Could you check a few things on this model? Use its own coordinates, in mm. A direction names the side the tool comes from. Coordinates: 2 decimals unless noted, no trailing zeros. Loops run counter-clockwise (first coordinate to the right, second up) from the corner with the lowest first, then second, coordinate; pieces in that order, holes last.
1) Imagine slicing it at B-B on x = -11.25. Please give me the cut outline in (y, z) (3 decimals).
2) Will these pins go through, and if not, where does the flat tip stop? P1, Ø8, axis at y = 51, z = 36, coming from the +X side; P2, Ø3, axis at y = 14, z = 65.5, coming from the -X side; P3, Ø8, axis at y = 56.5, z = 43, coming from the +X side.
3) If I drill on line 1 along Y through (x, z) = (-6.75, 43); line 2 along Y through (x, z) = (2.25, 12.5); line 3 along Y through (x, z) = (-6.5, 71), over which ranges is the centre line in solid material (lowest first)?
4) Imagine slicing it at A-A on y = 58. Please give me the cut outline in (x, z), plus the area to 3 significant figures.
5) Imagine slicing it at C-C on y = 26. Give the number of separate pieces and of enclosed holes in the cut face, plus the area to 3 significant figures.
6) For faces 3 (the face through (3.048, 25, 37)), 4 (the face through (-2, 19, 57.023)), which set-ups out of +Z, -Z, +X, -X, +Y, -Y let a thin tool reach every point of the face, with its end or its side?
7) Thinking about a two-plate mould opening in Z: for faces 1 (the face through (-2, 19, 2.159)), 2 (the face through (2, 0, 55)), which applies, released by +Z, released by -Z, zero draft, split by the parting line, or undercut?
```python
from build123d import *

# Parameters (mm, degrees)
BOSS_EXTRUDE1_DEPTH = 75.184
FILLET1_R           = 6.35
SKETCH6_R           = 3.175
CUT_EXTRUDE2_DEPTH  = 62.992
SKETCH11_W          = 5.969
SKETCH11_H          = 31.75
CUT_EXTRUDE6_DEPTH  = 100.663851822


with BuildPart() as part:
    # Sketch1 → Boss-Extrude1 (new body)
    with BuildSketch(Plane.XY):
        Polygon((0, 0), (3.048, 0), (3.048, 41.91), (-6.35, 47.752), (-6.35, 63.5), (-12.7, 63.5), (-12.7, 40.64), align=None)
    extrude(amount=BOSS_EXTRUDE1_DEPTH)

    # Fillet1
    fillet1_edges = [part.edges().sort_by_distance(p)[0] for p in [
        (-9.525, 63.5, 75.184),
        (-9.525, 63.5, 0),
    ]]
    fillet(fillet1_edges, radius=FILLET1_R)

    # Sketch6 → Cut-Extrude2 (cut, symmetric)
    with BuildSketch(Plane(origin=(-6.35, 0, 0), x_dir=(0, 0, -1), z_dir=(1, 0, 0))):
        with Locations(Location((-68.834, 57.15, 0), (0, 0, 90))):
            Circle(SKETCH6_R)
        with Locations(Location((-6.35, 57.15, 0), (0, 0, 90))):
            Circle(SKETCH6_R)
    extrude(amount=CUT_EXTRUDE2_DEPTH, both=True, mode=Mode.SUBTRACT)

    # Sketch11 → Cut-Extrude6 (cut, through all)
    with BuildSketch(Plane(origin=(3.048, 0, 0), x_dir=(0, 0, -1), z_dir=(1, 0, 0))):
        with Locations((-69.1515, 15.875)):
            Rectangle(SKETCH11_W, SKETCH11_H)
        with Locations((-60.0075, 15.875)):
            Rectangle(SKETCH11_W, SKETCH11_H)
        with Locations((-50.8635, 15.875)):
            Rectangle(SKETCH11_W, SKETCH11_H)
        with Locations((-41.7195, 15.875)):
            Rectangle(SKETCH11_W, SKETCH11_H)
        with Locations((-32.5755, 15.875)):
            Rectangle(SKETCH11_W, SKETCH11_H)
        with Locations((-23.4315, 15.875)):
            Rectangle(SKETCH11_W, SKETCH11_H)
        with Locations((-14.2875, 15.875)):
            Rectangle(SKETCH11_W, SKETCH11_H)
        with Locations((-5.1435, 15.875)):
            Rectangle(SKETCH11_W, SKETCH11_H)
    extrude(amount=-CUT_EXTRUDE6_DEPTH, mode=Mode.SUBTRACT)


solid = part.part
```
Filled in:
1. outline: (36, 0) - (57.15, 0) arc R6.35 ccw to (63.5, 6.35) - (63.5, 68.834) arc R6.35 ccw to (57.15, 75.184) - (36, 75.184) - close; hole circle Ø6.35 at (57.15, 6.35); hole circle Ø6.35 at (57.15, 68.834)
2. P1: stops at x = -5.14
2. P2: stops at x = -4.84
2. P3: stops at x = -6.35
3. line 1: y = 31.75 to 63.5
3. line 2: y = 31.75 to 42.41
3. line 3: y = 31.75 to 54.83, 59.47 to 63.12
4. outline: (-12.7, 0.06) - (-6.35, 0.06) - (-6.35, 3.29) - (-12.7, 3.29) - close; (-12.7, 9.41) - (-6.35, 9.41) - (-6.35, 65.77) - (-12.7, 65.77) - close; (-12.7, 71.89) - (-6.35, 71.89) - (-6.35, 75.13) - (-12.7, 75.13) - close
4. area: 399 mm2
5. separate pieces: 9
5. enclosed holes: 0
5. area: 306 mm2
6. face 3: +Z, -Z, +X, +Y, -Y
6. face 4: +X, -X, -Y
7. face 1: undercut
7. face 2: zero draft
